Answer from the drawing. Dimensions are ordinates in mm from the lowest x, y and z of the part. A direction names the side the tool comes from. Round coordinates to 2 decimals unless told otherwise and drop trailing zeros. Loops run counter-clockwise (first coordinate to the right, second up) from the corner with the lowest first, then second, coordinate; pieces in that order, holes last.
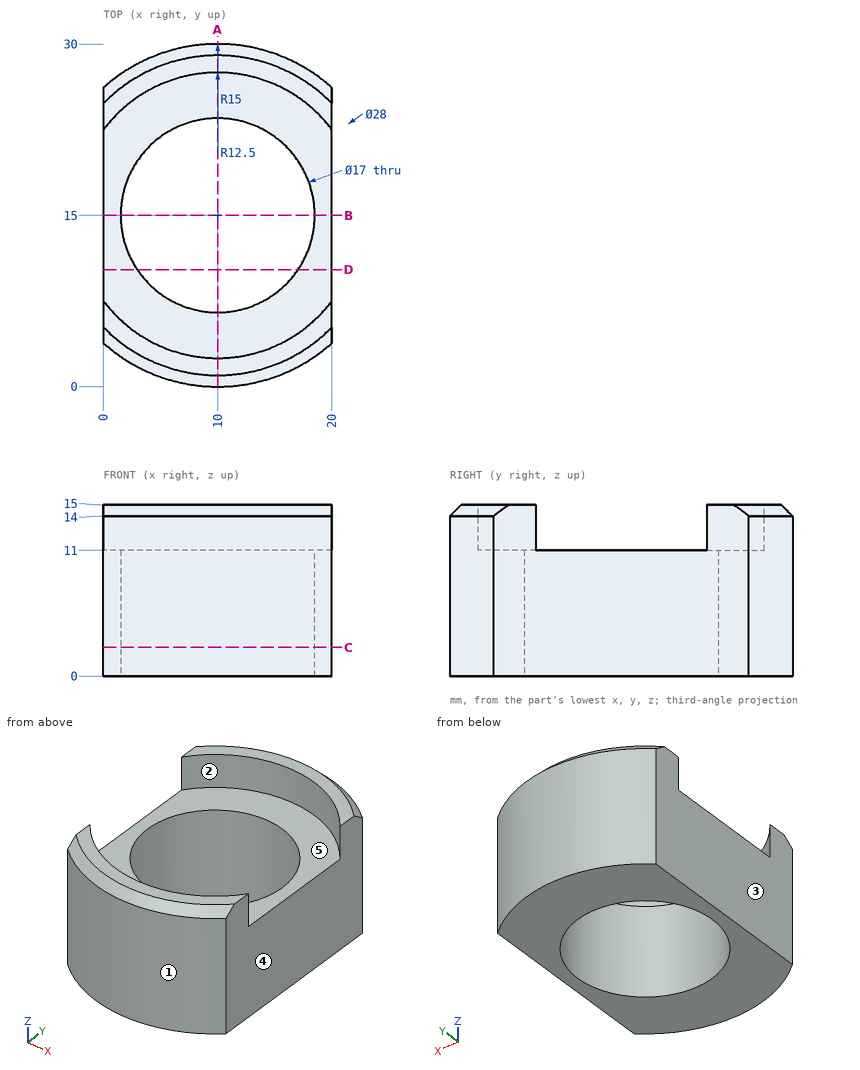
Item 1: Section C-C, the plane z = 2.5 is taken. Give the vertices of the cut face in (x, y), plus the area to 3 significant figures.
Item 2: Section D-D, the plane y = 10.25 is taken. Give the vertices of the cut face in (x, z), plus the area to 3 significant figures.
Item 3: Section A-A, the plane x = 10 is taken. Give the vertices of the cut face in (y, z), plus the area to 3 significant figures.
Item 4: Straight lines are drawn through the part: line 1 (Y direction, x = 10, z = 8.25); line 2 (Z direction, x = 8.5, y = 27); line 3 (Y direction, x = 19.25, z = 11.5). For each, find the intervals that lie inside material, in ascending order.
Item 5: Each of these flat-tipped pins is pushed along its axis until it touches: P1, Ø1.5, axis at x = 16, z = 8.5, coming from the +Y side; P2, Ø6, axis at x = 15, z = 3.5, coming from the -Y side; P3, Ø4, axis at y = 9.5, z = 12.5, coming from the +X side; P4, Ø2, axis at x = 7.5, z = 8, coming from the +Y side. Where does it stop, or does it pass through?
Item 6: Section B-B, the plane y = 15 is taken. Give the vertices of the cut face in (x, z).
Item 7: For the marked faces 4 and 5, determine the directions among +Z, -Z, +X, -X, +Y, -Y from which every point of the face is accessible in a straight line to the end or side of a thin tool.
Item 8: Determine the mould class of the marked faces 1, 2 and 3 for opening direction Y: pulls with the +Y half, pulls with the -Y half, needs draft (parallel to the pull), parting line crosses it, or undercut.
Answer below:
1. outline: (0, 3.82) arc R15 ccw to (20, 3.82) - (20, 26.18) arc R15 ccw to (0, 26.18) - close; hole circle Ø17 at (10, 15)
1. area: 325 mm2
2. outline: (0, 0) - (2.95, 0) - (2.95, 11) - (0, 11) - close; (17.05, 0) - (20, 0) - (20, 11) - (17.05, 11) - close
2. area: 64.9 mm2
3. outline: (0, 0) - (6.5, 0) - (6.5, 11) - (2.5, 11) - (2.5, 15) - (1, 15) - (0, 14) - close; (23.5, 0) - (30, 0) - (30, 14) - (29, 15) - (27.5, 15) - (27.5, 11) - (23.5, 11) - close
3. area: 162 mm2
4. line 1: y = 0 to 6.5, 23.5 to 30
4. line 2: z = 0 to 11
4. line 3: y = 3.19 to 6.59, 23.41 to 26.81
5. P1: stops at y = 29.05
5. P2: stops at y = 0.13
5. P3: stops at x = 20
5. P4: stops at y = 29.92
6. outline: (0, 0) - (1.5, 0) - (1.5, 11) - (0, 11) - close; (18.5, 0) - (20, 0) - (20, 11) - (18.5, 11) - close
7. face 4: +Z, -Z, +X, +Y, -Y
7. face 5: +Z
8. face 1: pulls with the -Y half
8. face 2: undercut
8. face 3: needs draft
